Here's the drawing with two shaded views (mm, measured from the low corner). I have some questions. A direction names the side the tool comes from. Coordinates: 2 decimals unless noted, no trailing zeros. Loops run counter-clockwise (first coordinate to the right, second up) from the corner with the lowest first, then second, coordinate; pieces in that order, holes last. Notation, with made-up numbers: (10, 87) -> (57, 87) arc R20 ccw to (57, 95) -> close; hole circle Ø5 at (78.25, 21.25). An arc over 180 degrees is marked (long way). Answer as a JSON object with one key per item and string values. Group by question number.
1) I'm going to push flat-ended pins straight in: pin 1 (4 mm diameter, centred on y = 31, z = 7, fed in from -X); pin 2 (1.5 mm diameter, centred on y = 27.5, z = 1.5, fed in from -X); pin 3 (3 mm diameter, centred on x = 8, y = 27.5, fed in from -Z); pin 4 (3 mm diameter, centred on x = 12, z = 2, fed in from -Y). Where does each tip first touch, or does it pass through?
2) I need wall thicknesses on probe 1 along X at (y, z) = (17, 6.5); probe 2 along Z at (x, y) = (28.5, 24.5); probe 3 along Y at (x, z) = (17.5, 4.5). Which ranges of each line are inside material? Lowest first, please. Write a range as [from, to].
3) I want a section at A-A (z = 5.25). Write out the boundary of the cut face in (x, y), then the cut area to 3 significant figures.
4) Which directions (+Z, -Z, +X, -X, +Y, -Y) give clear straight access to the entire face, cutting with the end or side of a thin tool? Please do the marked faces 1, 2 and 3.
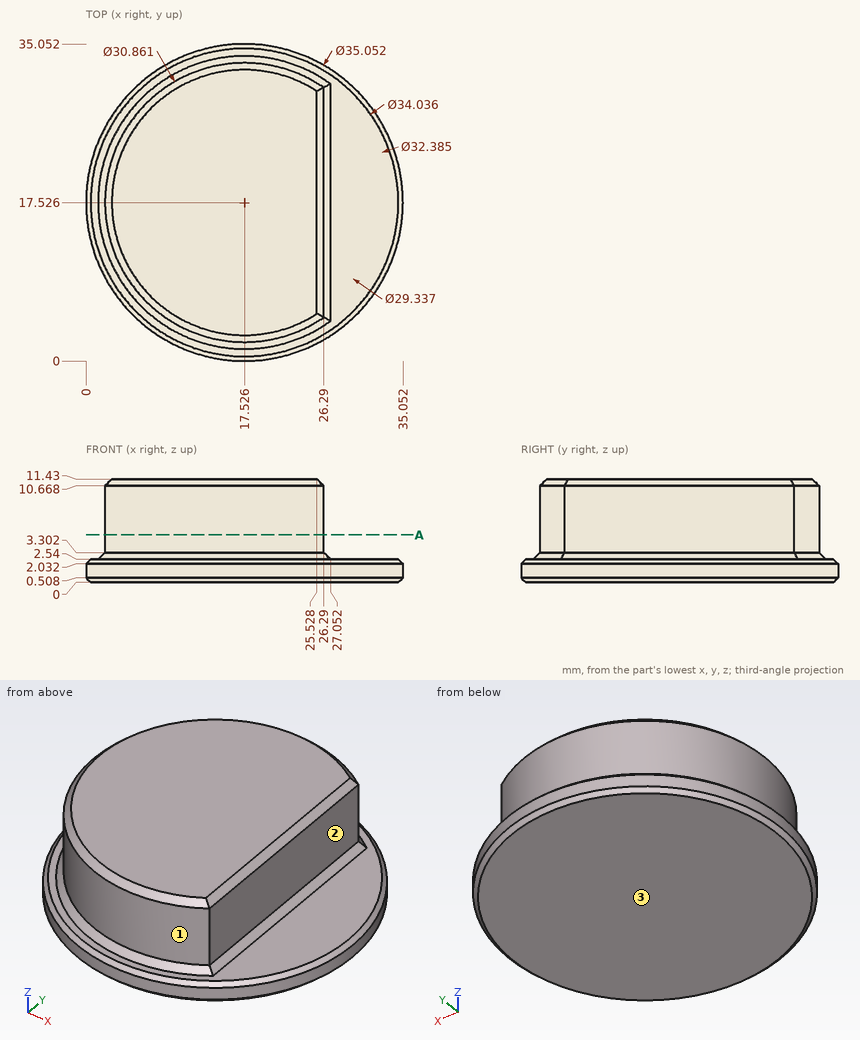
Determined:
{
 "1": {"pin 1": "x = 7.21", "pin 2": "x = 2.62", "pin 3": "z = 0", "pin 4": "y = 0.47"},
 "2": {"probe 1": "[2.1, 26.29]", "probe 2": "[0, 2.54]", "probe 3": "[2.1, 32.96]"},
 "3": {"outline": "(26.29, 4.83) -> (26.29, 30.23) arc R15.43 ccw (long way) to start", "area": "629 mm^2"},
 "4": {"face 1": "+Z", "face 2": "+Z, +X, +Y, -Y", "face 3": "-Z, +X, -X, +Y, -Y"}
}
